from build123d import *

# Parameters (mm, degrees)
SKETCH1_W           = 124
SKETCH1_H           = 64
BOSS_EXTRUDE1_DEPTH = 5
CUT_EXTRUDE1_DEPTH  = 5
SKETCH3_W           = 30.202540726
SKETCH3_H           = 30.202540726
CUT_EXTRUDE2_DEPTH  = 2
SKETCH4_R           = 2
CUT_EXTRUDE3_DEPTH  = 2
SKETCH5_R           = 8.025
SKETCH5_R_2         = 4.05
SKETCH5_R_3         = 25.5
CUT_EXTRUDE4_DEPTH  = 5
SKETCH6_R           = 1.25
CUT_EXTRUDE5_DEPTH  = 10
FILLET1_R           = 3
FILLET2_R           = 1.5
SKETCH7_R           = 9
CUT_EXTRUDE6_DEPTH  = 0.8
SKETCH8_R           = 1.25
CUT_EXTRUDE7_DEPTH  = 5


with BuildPart() as part:
    # Sketch1 → Boss-Extrude1 (new body)
    with BuildSketch(Plane(origin=(0, 0, 0), x_dir=(1, 0, 0), z_dir=(0, 1, 0))):
        with Locations((62, -32)):
            Rectangle(SKETCH1_W, SKETCH1_H)
    extrude(amount=BOSS_EXTRUDE1_DEPTH)

    # Sketch2 → Cut-Extrude1 (cut)
    with BuildSketch(Plane(origin=(0, 5, 0), x_dir=(1, 0, 0), z_dir=(0, 1, 0))):
        with BuildLine():
            Line((15.897459274, -12.997459274), (15.897459274, 12.365379101))
            Line((15.897459274, 12.365379101), (28.097459274, 12.365379101))
            Line((28.097459274, 12.365379101), (28.097459274, -12.997459274))
            ThreePointArc((28.097459274, -12.997459274), (21.997459274, -19.097459274), (15.897459274, -12.997459274))
        make_face()
        with BuildLine():
            Line((95.902540726, 12.365379101), (95.902540726, -12.997459274))
            ThreePointArc((95.902540726, -12.997459274), (102.002540726, -19.097459274), (108.102540726, -12.997459274))
            Line((108.102540726, -12.997459274), (108.102540726, 12.365379101))
            Line((108.102540726, 12.365379101), (95.902540726, 12.365379101))
        make_face()
    extrude(amount=-CUT_EXTRUDE1_DEPTH, mode=Mode.SUBTRACT)

    # Sketch3 → Cut-Extrude2 (cut)
    with BuildSketch(Plane.XZ):
        with Locations((18.998729637, 44.998729637)):
            Rectangle(SKETCH3_W, SKETCH3_H)
        with Locations((105.001270363, 44.998729637)):
            Rectangle(SKETCH3_W, SKETCH3_H)
    extrude(amount=-CUT_EXTRUDE2_DEPTH, mode=Mode.SUBTRACT)

    # Sketch4 → Cut-Extrude3 (cut)
    with BuildSketch(Plane.XZ):
        with Locations((34.1, 29.897459274)):
            Circle(SKETCH4_R)
        with Locations((34.1, 60.1)):
            Circle(SKETCH4_R)
        with Locations((3.897459274, 60.1)):
            Circle(SKETCH4_R)
        with Locations((3.897459274, 29.897459274)):
            Circle(SKETCH4_R)
        with Locations((120.102540726, 29.897459274)):
            Circle(SKETCH4_R)
        with Locations((120.102540726, 60.1)):
            Circle(SKETCH4_R)
        with Locations((89.9, 60.1)):
            Circle(SKETCH4_R)
        with Locations((89.9, 29.897459274)):
            Circle(SKETCH4_R)
    extrude(amount=-CUT_EXTRUDE3_DEPTH, mode=Mode.SUBTRACT)

    # Sketch5 → Cut-Extrude4 (cut)
    with BuildSketch(Plane(origin=(0, 5, 0), x_dir=(1, 0, 0), z_dir=(0, 1, 0))):
        with Locations(Location((62, -21.148702719, 0), (0, 0, 270))):
            Circle(SKETCH5_R)
        with Locations(Location((18.998729637, -44.998729637, 0), (0, 0, 270))):
            Circle(SKETCH5_R_2)
        with Locations(Location((105.001270363, -44.998729637, 0), (0, 0, 270))):
            Circle(SKETCH5_R_2)
        with Locations((62, -76.5)):
            Circle(SKETCH5_R_3)
    extrude(amount=-CUT_EXTRUDE4_DEPTH, mode=Mode.SUBTRACT)

    # Sketch6 → Cut-Extrude5 (cut)
    with BuildSketch(Plane(origin=(0, 5, 0), x_dir=(1, 0, 0), z_dir=(0, 1, 0))):
        with Locations(Location((92.002540726, -19.497459274, 0), (0, 0, 270))):
            Circle(SKETCH6_R)
        with Locations(Location((112.002540726, -19.497459274, 0), (0, 0, 270))):
            Circle(SKETCH6_R)
        with Locations(Location((31.997459274, -19.497459274, 0), (0, 0, 270))):
            Circle(SKETCH6_R)
        with Locations(Location((11.997459274, -19.497459274, 0), (0, 0, 270))):
            Circle(SKETCH6_R)
    extrude(amount=-CUT_EXTRUDE5_DEPTH, mode=Mode.SUBTRACT)

    # Fillet1
    fillet1_edges = [part.edges().sort_by_distance(p)[0] for p in [
        (0, 2.5, 0),
        (124, 2.5, 0),
        (124, 2.5, 64),
        (0, 2.5, 64),
    ]]
    fillet(fillet1_edges, radius=FILLET1_R)

    # Fillet2
    fillet2_edges = [part.edges().sort_by_distance(p)[0] for p in [
        (39.773889229, 2.5, 64),
        (84.226110771, 2.5, 64),
        (15.897459274, 2.5, 0),
        (28.097459274, 2.5, 0),
        (95.902540726, 2.5, 0),
        (108.102540726, 2.5, 0),
    ]]
    fillet(fillet2_edges, radius=FILLET2_R)

    # Sketch7 → Cut-Extrude6 (cut)
    with BuildSketch(Plane(origin=(0, 5, 0), x_dir=(1, 0, 0), z_dir=(0, 1, 0))):
        with Locations(Location((62, -21.148702719, 0), (0, 0, 270))):
            Circle(SKETCH7_R)
    extrude(amount=-CUT_EXTRUDE6_DEPTH, mode=Mode.SUBTRACT)

    # Sketch8 → Cut-Extrude7 (cut)
    with BuildSketch(Plane(origin=(0, 5, 0), x_dir=(1, 0, 0), z_dir=(0, 1, 0))):
        with Locations(Location((51, -21.148702719, 0), (0, 0, 270))):
            Circle(SKETCH8_R)
        with Locations(Location((73, -21.148702719, 0), (0, 0, 90))):
            Circle(SKETCH8_R)
    extrude(amount=-CUT_EXTRUDE7_DEPTH, mode=Mode.SUBTRACT)


solid = part.part
Check sheet for the modelled part. Datum: model origin and axes. Units: mm. A direction names the side the tool comes from. Give positions to 0.01 mm unless a question says otherwise; leave off trailing zeros. Loops run counter-clockwise (first coordinate to the right, second up) from the corner with the lowest first, then second, coordinate; pieces in that order, holes last. Notation, with made-up numbers: M -23.75,-17 L -0.75,-17 A19 ccw -0.75,-5 Z; hole C 0,10.5 d7. An arc over 180 degrees is marked long. Return JSON: item names as keys, results as strings. Group by question number.
1. Mould release check, pull along Z, two halves, no side actions. Record for faces 6 (the flat face through (103, 2, 64)), 7 (the cylindrical face through (88.44, 0.99, 28.53)), 8 (the cylindrical face through (0.86, 2.54, 0.9)): released by +Z, released by -Z, zero draft, split by the parting line, or undercut.
2. Cross-section at A-A on x = 62. Record the boundary of the cut face in (y, z), plus the area to 3 significant figures.
3. Thickness scan on L1, parallel to X at y = 3.9, z = 9.5; L2, parallel to X at y = 0.7, z = 43; L3, parallel to Y at x = 67.5, z = 28. Record the ranges inside material, lowest first.
4. Cross-section at C-C on z = 56.5. Record the boundary of the cut face in (x, y), plus the area to 3 significant figures.
5. Tool access check on faces 1 (the cylindrical face through (113.24, 2.54, 19.33)), 2 (the flat face through (95.903, 3, 7)), 3 (the cylindrical face through (2.44, 0.99, 28.53)), 4 (the cylindrical face through (123.14, 2.54, 0.9)), 5 (the cylindrical face through (53.214, 4.606, 19.198)). Record the directions out of +Z, -Z, +X, -X, +Y, -Y that give a thin tool (end or side, any length) a straight path to the whole face; none if there is none.
6. Cross-section at D-D on z = 43.5. Record the boundary of the cut face in (x, y).
7. Cross-section at B-B on z = 34. Record the boundary of the cut face in (x, y), plus the area to 3 significant figures.
8. Go/stop test with flat-tipped pins: pin 1 (2 mm diameter, centred on x = 92, z = 19.5, fed in from -Y); pin 2 (1 mm diameter, centred on x = 15, y = 1, fed in from -Z); pin 3 (10.5 mm diameter, centred on x = 105, z = 45, fed in from -Y); pin 4 (4 mm diameter, centred on x = 112, z = 19.5, fed in from +Y). Record where each tip stops, or that it passes through.
Return value:
{
 "1": {"face 6": "released by +Z", "face 7": "undercut", "face 8": "released by -Z"},
 "2": {"outline": "M 0,0 L 5,0 L 5,12.15 L 4.2,12.15 L 4.2,13.12 L 0,13.12 Z; M 0,29.17 L 4.2,29.17 L 4.2,30.15 L 5,30.15 L 5,51 L 0,51 Z", "area": "173 mm^2"},
 "3": {"L1": "0 to 15.9, 28.1 to 95.9, 108.1 to 124", "L2": "0 to 3.9, 34.1 to 89.9, 120.1 to 124", "L3": "0 to 4.2"},
 "4": {"outline": "M 0,0 L 3.9,0 L 3.9,2 L 34.1,2 L 34.1,0 L 46.18,0 L 46.18,5 L 0,5 Z; M 77.82,0 L 89.9,0 L 89.9,2 L 120.1,2 L 120.1,0 L 124,0 L 124,5 L 77.82,5 Z", "area": "341 mm^2"},
 "5": {"face 1": "+Y, -Y", "face 2": "-Z, +Y, -Y", "face 3": "-Y", "face 4": "-Z, +X, +Y, -Y", "face 5": "+Y"},
 "6": {"outline": "M 0,0 L 3.9,0 L 3.9,2 L 15.24,2 L 15.24,5 L 0,5 Z; M 22.76,2 L 34.1,2 L 34.1,0 L 89.9,0 L 89.9,2 L 101.24,2 L 101.24,5 L 22.76,5 Z; M 108.76,2 L 120.1,2 L 120.1,0 L 124,0 L 124,5 L 108.76,5 Z"},
 "7": {"outline": "M 0,0 L 3.9,0 L 3.9,2 L 34.1,2 L 34.1,0 L 89.9,0 L 89.9,2 L 120.1,2 L 120.1,0 L 124,0 L 124,5 L 0,5 Z", "area": "499 mm^2"},
 "8": {"pin 1": "through", "pin 2": "z = 0", "pin 3": "y = 2", "pin 4": "y = 5"}
}
